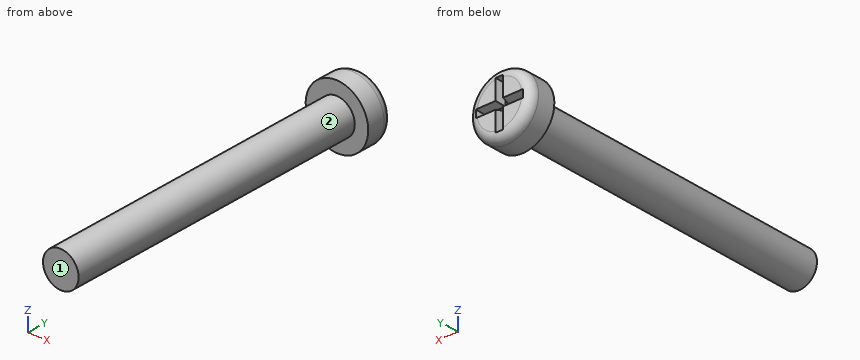
```python
from build123d import *

# Parameters (mm, degrees)
SKETCH_1_R          = 2
EXTRUDE_1_DEPTH     = 35
SKETCH_2_R          = 3.515
EXTRUDE_2_DEPTH     = 3
CUT_EXTRUDE_1_DEPTH = 1
CUT_EXTRUDE_1_DRAFT = -12
FILLET_2_R          = 1


with BuildPart() as part:
    # Эскиз1 → Бобышка-Вытянуть1 (new body)
    with BuildSketch(Plane(origin=(0, 0, 0), x_dir=(1, 0, 0), z_dir=(0, 1, 0))):
        with Locations(Location((0, 0, 0), (0, 0, 270))):
            Circle(SKETCH_1_R)
    extrude(amount=EXTRUDE_1_DEPTH)

    # Эскиз2 → Бобышка-Вытянуть2 (add)
    with BuildSketch(Plane(origin=(0, 35, 0), x_dir=(1, 0, 0), z_dir=(0, 1, 0))):
        with Locations(Location((0, 0, 0), (0, 0, 270))):
            Circle(SKETCH_2_R)
    extrude(amount=EXTRUDE_2_DEPTH)


with BuildPart() as cut_extrude_1_tool:
    # Эскиз3 → Вырез-Вытянуть1 (with draft: the straight prism first)
    with BuildSketch(Plane(origin=(0, 38, 0), x_dir=(1, 0, 0), z_dir=(0, 1, 0))):
        Polygon((-2.641549473, 0.422769916), (-2.641549473, -0.422769916), (-0.422769916, -0.422769916), (-0.422769916, -2.641549473), (0.422769916, -2.641549473), (0.422769916, -0.422769916), (2.641549473, -0.422769916), (2.641549473, 0.422769916), (0.422769916, 0.422769916), (0.422769916, 2.641549473), (-0.422769916, 2.641549473), (-0.422769916, 0.422769916), align=None)
    extrude(amount=-CUT_EXTRUDE_1_DEPTH)
    # Вырез-Вытянуть1: the draft: its side faces are tilted about the plane it starts from
    cut_extrude_1_sides = [cut_extrude_1_tool.faces().sort_by_distance(p)[0] for p in [
        (-2.641549473, 37.5, 0),
        (-1.532159694, 37.5, 0.422769916),
        (-0.422769916, 37.5, 1.532159694),
        (0, 37.5, 2.641549473),
        (0.422769916, 37.5, 1.532159694),
        (1.532159694, 37.5, 0.422769916),
        (2.641549473, 37.5, 0),
        (1.532159694, 37.5, -0.422769916),
        (0.422769916, 37.5, -1.532159694),
        (0, 37.5, -2.641549473),
        (-0.422769916, 37.5, -1.532159694),
        (-1.532159694, 37.5, -0.422769916),
    ]]
    draft(cut_extrude_1_sides, Plane(origin=(0, 38, 0), x_dir=(1, 0, 0), z_dir=(0, 1, 0)), CUT_EXTRUDE_1_DRAFT)


with BuildPart() as part_1:
    add(part.part)

    # Вырез-Вытянуть1: cut by cut_extrude_1_tool
    add(cut_extrude_1_tool.part, mode=Mode.SUBTRACT)

    # Скругление2
    # the kernel refuses this fillet: 1 mm, written as the material it takes off along each edge
    with BuildSketch(Plane(origin=(0, 38, 0), x_dir=(0, 0, 1), z_dir=(-1, 0, 0))) as fillet_2_piece_1:
        with BuildLine():
            CenterArc((3.515 - FILLET_2_R, -FILLET_2_R), FILLET_2_R, 0, 90)
            Line((3.515 - FILLET_2_R, 0), (3.515, 0))
            Line((3.515, 0), (3.515, -FILLET_2_R))
        make_face()
    revolve(axis=Axis((0, 38, 0), (0, 1, 0)), mode=Mode.SUBTRACT)


solid = part_1.part
```
Verification items for the finished model (mm, model axes). Face numbers are marked on the shaded views. A direction names the side the tool comes from. Give positions to 0.01 mm unless a question says otherwise; leave off trailing zeros. Order: outer loops, then holes, each group sorted by start corner. A loop starts at its lowest first (then second) coordinate and runs counter-clockwise, first axis right, second up. Notation, with made-up numbers: (51, -35.5) -> (86, -35.5) arc R30 ccw to (86, -11.5) -> close; hole circle Ø11 at (88, -33.75). An arc over 180 degrees is marked (long way). One line per item, written item: value.
(1) Gauge pin test, flat ends, axial feed: pin 1 (2 mm diameter, centred on y = 12, z = 0.5, fed in from +X); pin 2 (4 mm diameter, centred on y = 32.5, z = -1.5, fed in from -X). Record the tip position at first contact, or that the pin passes through.
Final values:
pin 1: x = 2
pin 2: x = -2
(2) Tool access check on the marked faces 1 and 2. Record the directions out of +Z, -Z, +X, -X, +Y, -Y that give a thin tool (end or side, any length) a straight path to the whole face; none if there is none.
Final values:
face 1: +Z, -Z, +X, -X, -Y
face 2: -Y
(3) Scan lines: line 1 along Y through (x, z) = (1.75, -1.5); line 2 along Y through (x, z) = (1.25, 0); line 3 along X through (y, z) = (5, -1). Record each from-to range of solid material in increasing order. Write a range as [from, to].
Final values:
line 1: [35, 38]
line 2: [0, 37]
line 3: [-1.73, 1.73]
(4) Sectioned sample at A-A on y = 9. Record the cut outline in (x, z).
Final values:
outline: circle Ø4 at (0, 0)
